from build123d import *

# Parameters (mm, degrees)
SKETCH1_R           = 19.05
SKETCH1_R_2         = 3.81
BOSS_EXTRUDE1_DEPTH = 5.08
SKETCH2_R           = 19.05
BOSS_EXTRUDE2_DEPTH = 5.08


with BuildPart() as part:
    # Sketch1 → Boss-Extrude1 (new body)
    with BuildSketch(Plane(origin=(0, 0, 0), x_dir=(0, 0, -1), z_dir=(1, 0, 0))):
        Circle(SKETCH1_R)
        Circle(SKETCH1_R_2, mode=Mode.SUBTRACT)
    extrude(amount=BOSS_EXTRUDE1_DEPTH)

    # Sketch2 → Boss-Extrude2 (add)
    with BuildSketch(Plane(origin=(5.08, 0, 0), x_dir=(0, 0, -1), z_dir=(1, 0, 0))):
        Circle(SKETCH2_R)
        Polygon((7.5, 0), (3.75, 6.495190528), (-3.75, 6.495190528), (-7.5, 0), (-3.75, -6.495190528), (3.75, -6.495190528), align=None, mode=Mode.SUBTRACT)
    extrude(amount=BOSS_EXTRUDE2_DEPTH)


solid = part.part
Can you work these out from the model? Positions are in its coordinate system, mm. A direction names the side the tool comes from. Round coordinates to 2 decimals unless told otherwise and drop trailing zeros. Order: outer loops, then holes, each group sorted by start corner. A loop starts at its lowest first (then second) coordinate and runs counter-clockwise, first axis right, second up. Notation, with made-up numbers: M 69.25,64.5 L 110.25,64.5 A22 ccw 110.25,102.5 Z; hole C 60.25,15.5 d4. An arc over 180 degrees is marked long. Use a Markdown table: item, result.
1) Imagine slicing it at D-D (z = 4.5). List the corners of the cut face in (x, y) for me.
Geometry says:
| item | result |
|---|---|
| outline | M 0,-18.51 L 10.16,-18.51 L 10.16,-5.2 L 5.08,-5.2 L 5.08,5.2 L 10.16,5.2 L 10.16,18.51 L 0,18.51 Z |
2) I'm going to push flat-ended pins straight in: P1, Ø6.5, axis at y = -0.5, z = -1, coming from the +X side; P2, Ø1.5, axis at x = 6, z = -13.5, coming from the -Y side; P3, Ø1, axis at x = 3, z = 0, coming from the -Y side. Where does each tip first touch, or does it pass through?
Geometry says:
| item | result |
|---|---|
| P1 | stops at x = 5.08 |
| P2 | stops at y = -14.15 |
| P3 | stops at y = -19.05 |
3) Imagine slicing it at A-A (z = 0). List the corners of the cut face in (x, y) for me, then the cut area to 3 significant figures.
Geometry says:
| item | result |
|---|---|
| outline | M 0,-19.05 L 10.16,-19.05 L 10.16,-6.5 L 5.08,-6.5 L 5.08,-3.81 L 0,-3.81 Z; M 0,3.81 L 5.08,3.81 L 5.08,6.5 L 10.16,6.5 L 10.16,19.05 L 0,19.05 Z |
| area | 282 mm² |
4) Imagine slicing it at B-B (x = 6.5). List the corners of the cut face in (y, z) for me.
Geometry says:
| item | result |
|---|---|
| outline | C 0,0 d38.1; hole M -6.5,-3.75 L 0,-7.5 L 6.5,-3.75 L 6.5,3.75 L 0,7.5 L -6.5,3.75 Z |
5) On a 3-axis mill with a long thin cutter (end or side, diameter ignored), from which of +Z, -Z, +X, -X, +Y, -Y can I reach the whole of each face in a straight line? I mean faces 5 (the face through (8, -6.495, 0)), 6 (the face through (2.5, -3.72, 0.83)). Say none if no direction works.
Geometry says:
| item | result |
|---|---|
| face 5 | +X |
| face 6 | +X, -X |
6) Imagine slicing it at C-C (x = 2.75). List the corners of the cut face in (y, z) for me.
Geometry says:
| item | result |
|---|---|
| outline | C 0,0 d38.1; hole C 0,0 d7.62 |
7) If I drill on line 1 along Y through (x, z) = (3.75, 0); line 2 along X through (y, z) = (-0.5, -6.5); line 3 along Z through (x, y) = (1.25, 2), over which ranges is the centre line in solid material (lowest first)?
Geometry says:
| item | result |
|---|---|
| line 1 | y = -19.05 to -3.81, 3.81 to 19.05 |
| line 2 | x = 0 to 5.08 |
| line 3 | z = -18.94 to -3.24, 3.24 to 18.94 |
8) If we mould it in two halves opening along Z, with no side actions, what happens to faces 1 (the face through (5.01, -11.59, 15.12)), 2 (the face through (7.584, -3.202, 5.651)), 3 (the face through (5.08, 3, -3)), 4 (the face through (10.16, 0, -8))? For each: +Z half, -Z half, draft (parallel to the pull), parting line (faces both ways), or undercut.
Geometry says:
| item | result |
|---|---|
| face 1 | parting line |
| face 2 | undercut |
| face 3 | undercut |
| face 4 | draft |
